Geometry check sheet. Reference: the model listing, model coordinates, mm. A direction names the side the tool comes from. Round coordinates to 2 decimals unless told otherwise and drop trailing zeros. Order: outer loops, then holes, each group sorted by start corner. A loop starts at its lowest first (then second) coordinate and runs counter-clockwise, first axis right, second up.
(1) Draft check along X on faces 6 (the face through (-42, 0, 3.2)), 7 (the face through (-0.7, 0.1, 0)), 8 (the face through (-49, 0, 3.2)), 9 (the face through (37.4, 0, 2.7)). Enter one of: pulls with the +X half, pulls with the -X half, needs draft (parallel to the pull), parting line crosses it, or undercut.
(2) Gauge pin test, flat end, axial feed: P1, Ø1, axis at x = -42, y = 0.5, coming from the +Z side. Record the tip position at first contact, or that the pin passes through.
(3) Thickness scan on L1, parallel to X at y = 3, z = 3.35; L2, parallel to Z at x = 27.5, y = 0; L3, parallel to Y at x = 44, z = 3.95. Record the ranges inside material, lowest first.
(4) Cross-section at D-D on x = -2.5. Enter the section's corners in (y, z).
(5) Cross-section at C-C on x = -42.5. Enter the section's corners in (y, z).
(6) Cross-section at B-B on x = 27.5. Enter the section's corners in (y, z), and give its area (3 significant figures).
(7) Set-up check for faces 1 (the face through (-1, -4.5, 3)), 2 (the face through (-1, 0, 2)), 3 (the face through (46, -1.6, 3)), 4 (the face through (-41.32, 1.08, 4.11)), 5 (the face through (-1, 0, 5)): record each of +Z, -Z, +X, -X, +Y, -Y from which the full face is reachable in a straight line by a thin tool's end or side.
from build123d import *

# Parameters (mm, degrees)
SKETCH1_W           = 105
SKETCH1_H           = 9
BOSS_EXTRUDE1_DEPTH = 5
CUT_EXTRUDE1_DEPTH  = 5
SKETCH8_W           = 8
SKETCH8_H           = 3.2
CUT_EXTRUDE4_DEPTH  = 10
SKETCH7_R           = 3.25
SKETCH7_R_2         = 1.6
CUT_EXTRUDE2_DEPTH  = 1.8
CHAMFER1_SIZE       = 0.4
CHAMFER2_SIZE       = 0.4
SKETCH2_R           = 1.65
CUT_EXTRUDE3_DEPTH  = 10
SKETCH10_R          = 1.5
CUT_EXTRUDE5_DEPTH  = 4


with BuildPart() as part:
    # Sketch1 → Boss-Extrude1 (new body)
    with BuildSketch(Plane.XY):
        Rectangle(SKETCH1_W, SKETCH1_H)
    extrude(amount=BOSS_EXTRUDE1_DEPTH)

    # Sketch4 → Cut-Extrude1 (cut)
    with BuildSketch(Plane.XY.offset(5)):
        with BuildLine():
            Line((39, 1.6), (45, 1.6))
            ThreePointArc((45, 1.6), (46.6, 0), (45, -1.6))
            Line((45, -1.6), (39, -1.6))
            ThreePointArc((39, -1.6), (37.4, 0), (39, 1.6))
        make_face()
    extrude(amount=-CUT_EXTRUDE1_DEPTH, mode=Mode.SUBTRACT)

    # Sketch8 → Cut-Extrude4 (cut)
    with BuildSketch(Plane.XY.offset(5)):
        with Locations((48.5, 0)):
            Rectangle(SKETCH8_W, SKETCH8_H)
    extrude(amount=-CUT_EXTRUDE4_DEPTH, mode=Mode.SUBTRACT)

    # Sketch7 → Cut-Extrude2 (cut)
    with BuildSketch(Plane(origin=(0, 0, 5), x_dir=(-1, 0, 0), z_dir=(0, 0, -1))):
        with Locations((48.85, 0)):
            Circle(SKETCH7_R)
        with Locations((42.5, 0)):
            Circle(SKETCH7_R_2)
    extrude(amount=CUT_EXTRUDE2_DEPTH, mode=Mode.SUBTRACT)

    # Chamfer1
    chamfer1_edges = [part.edges().sort_by_distance(p)[0] for p in [
        (-45.6, 0, 5),
    ]]
    chamfer(chamfer1_edges, length=CHAMFER1_SIZE - 0.0001)  # a hair under: the kernel refuses the full size

    # Chamfer2
    chamfer2_edges = [part.edges().sort_by_distance(p)[0] for p in [
        (37.4, 0, 0),
        (45.75, 1.6, 0),
        (45.75, -1.6, 0),
        (52.5, 3.05, 0),
        (0, 4.5, 0),
        (52.5, -3.05, 0),
        (0, -4.5, 0),
        (-52.5, 0, 0),
    ]]
    chamfer(chamfer2_edges, length=CHAMFER2_SIZE)

    # Sketch2 → Cut-Extrude3 (cut)
    with BuildSketch(Plane(origin=(0, 4.5, 0), x_dir=(1, 0, 0), z_dir=(0, 1, 0))):
        with Locations(Location((27.5, -2.5, 0), (0, 0, 180))):
            Circle(SKETCH2_R)
    extrude(amount=-CUT_EXTRUDE3_DEPTH, mode=Mode.SUBTRACT)

    # Sketch10 → Cut-Extrude5 (cut, symmetric)
    with BuildSketch(Plane.XY):
        with Locations((-2.5, 0)):
            Circle(SKETCH10_R)
    extrude(amount=CUT_EXTRUDE5_DEPTH, both=True, mode=Mode.SUBTRACT)


solid = part.part
Found:
1. face 6: undercut
1. face 7: needs draft
1. face 8: undercut
1. face 9: pulls with the +X half
2. P1: stops at z = 3.2
3. L1: x = -52.5 to -50.1, -47.6 to 26.09, 28.91 to 52.5
3. L2: z = 0 to 0.85, 4.15 to 5
3. L3: y = -4.5 to -1.6, 1.6 to 4.5
4. outline: (-4.5, 0.4) - (-4.1, 0) - (-1.5, 0) - (-1.5, 4) - (1.5, 4) - (1.5, 0) - (4.1, 0) - (4.5, 0.4) - (4.5, 5) - (-4.5, 5) - close
5. outline: (-4.5, 0.4) - (-4.1, 0) - (4.1, 0) - (4.5, 0.4) - (4.5, 5) - (1.6, 5) - (1.6, 3.2) - (-1.6, 3.2) - (-1.6, 5) - (-4.5, 5) - close
6. outline: (-4.5, 0.4) - (-4.1, 0) - (4.1, 0) - (4.5, 0.4) - (4.5, 0.85) - (-4.5, 0.85) - close; (-4.5, 4.15) - (4.5, 4.15) - (4.5, 5) - (-4.5, 5) - close
6. area: 15.1 mm2
7. face 1: +Z, -Z, +X, -X, -Y
7. face 2: -Z
7. face 3: +Z, -Z, +X
7. face 4: +Z
7. face 5: +Z, +X, -X, +Y, -Y
